from build123d import *

# Parameters (mm, degrees)
SKETCH_1_W          = 400
SKETCH_1_H          = 80
EXTRUDE_1_DEPTH     = 35
SKETCH_2_W          = 400
SKETCH_2_H          = 61
CUT_EXTRUDE_1_DEPTH = 10
CHAMFER_1_SIZE      = 5
CHAMFER_2_SIZE      = 10
CHAMFER_2_SIZE2     = 7.002075382
CHAMFER_3_SIZE      = 10
CHAMFER_3_SIZE2     = 7.002075382
CHAMFER_4_SIZE      = 10
CHAMFER_4_SIZE2     = 7.002075382
CHAMFER_5_SIZE      = 10
CHAMFER_5_SIZE2     = 7.002075382
CUT_EXTRUDE_2_REACH = 207.487
SKETCH_3_R          = 9
SKETCH_3_R_2        = 10


with BuildPart() as part:
    # 草图1 → 凸台-拉伸1 (new body)
    with BuildSketch(Plane.XY):
        Rectangle(SKETCH_1_W, SKETCH_1_H)
    extrude(amount=EXTRUDE_1_DEPTH)

    # 草图2 → 切除-拉伸1 (cut)
    with BuildSketch(Plane.XY.offset(35)):
        with Locations((0, 9.5)):
            Rectangle(SKETCH_2_W, SKETCH_2_H)
    extrude(amount=-CUT_EXTRUDE_1_DEPTH, mode=Mode.SUBTRACT)

    # 倒角1
    chamfer_1_edges = [part.edges().sort_by_distance(p)[0] for p in [
        (0, 40, 25),
        (0, 40, 0),
    ]]
    chamfer(chamfer_1_edges, length=CHAMFER_1_SIZE)

    # 倒角2
    chamfer_2_edges = [part.edges().sort_by_distance(p)[0] for p in [
        (0, -40, 35),
    ]]
    chamfer_2_side = [part.faces().sort_by_distance(p)[0] for p in [
        (0, -40, 17.5),
    ]]
    chamfer(chamfer_2_edges, length=CHAMFER_2_SIZE, length2=CHAMFER_2_SIZE2, reference=chamfer_2_side[0])

    # 倒角3
    chamfer_3_edges = [part.edges().sort_by_distance(p)[0] for p in [
        (0, -40, 0),
    ]]
    chamfer_3_side = [part.faces().sort_by_distance(p)[0] for p in [
        (0, -40, 12.5),
    ]]
    chamfer(chamfer_3_edges, length=CHAMFER_3_SIZE, length2=CHAMFER_3_SIZE2, reference=chamfer_3_side[0])

    # 倒角4
    chamfer_4_edges = [part.edges().sort_by_distance(p)[0] for p in [
        (-200, -40, 17.5),
    ]]
    chamfer_4_side = [part.faces().sort_by_distance(p)[0] for p in [
        (0, -40, 17.5),
    ]]
    chamfer(chamfer_4_edges, length=CHAMFER_4_SIZE, length2=CHAMFER_4_SIZE2, reference=chamfer_4_side[0])

    # 倒角5
    chamfer_5_edges = [part.edges().sort_by_distance(p)[0] for p in [
        (200, -40, 17.5),
    ]]
    chamfer_5_side = [part.faces().sort_by_distance(p)[0] for p in [
        (5, -40, 17.5),
    ]]
    chamfer(chamfer_5_edges, length=CHAMFER_5_SIZE, length2=CHAMFER_5_SIZE2, reference=chamfer_5_side[0])

    # 草图3 → 切除-拉伸2 (cut, up to next)
    with BuildSketch(Plane.XY.offset(25), mode=Mode.PRIVATE) as cut_extrude_2_sk1:
        with Locations((-150, 9.5)):
            Circle(SKETCH_3_R)
    cut_extrude_2_tool1 = extrude(cut_extrude_2_sk1.sketch, amount=-CUT_EXTRUDE_2_REACH, mode=Mode.PRIVATE) & part.part
    # 草图3 → 切除-拉伸2 (cut, up to next)
    with BuildSketch(Plane.XY.offset(25), mode=Mode.PRIVATE) as cut_extrude_2_sk2:
        with Locations((-100, 9.5)):
            Circle(SKETCH_3_R_2)
    cut_extrude_2_tool2 = extrude(cut_extrude_2_sk2.sketch, amount=-CUT_EXTRUDE_2_REACH, mode=Mode.PRIVATE) & part.part
    # 草图3 → 切除-拉伸2 (cut, up to next)
    with BuildSketch(Plane.XY.offset(25), mode=Mode.PRIVATE) as cut_extrude_2_sk3:
        with Locations((-50, 9.5)):
            Circle(SKETCH_3_R)
    cut_extrude_2_tool3 = extrude(cut_extrude_2_sk3.sketch, amount=-CUT_EXTRUDE_2_REACH, mode=Mode.PRIVATE) & part.part
    # 草图3 → 切除-拉伸2 (cut, up to next)
    with BuildSketch(Plane.XY.offset(25), mode=Mode.PRIVATE) as cut_extrude_2_sk4:
        with Locations((50, 9.5)):
            Circle(SKETCH_3_R)
    cut_extrude_2_tool4 = extrude(cut_extrude_2_sk4.sketch, amount=-CUT_EXTRUDE_2_REACH, mode=Mode.PRIVATE) & part.part
    # 草图3 → 切除-拉伸2 (cut, up to next)
    with BuildSketch(Plane.XY.offset(25), mode=Mode.PRIVATE) as cut_extrude_2_sk5:
        with Locations((100, 9.5)):
            Circle(SKETCH_3_R_2)
    cut_extrude_2_tool5 = extrude(cut_extrude_2_sk5.sketch, amount=-CUT_EXTRUDE_2_REACH, mode=Mode.PRIVATE) & part.part
    # 草图3 → 切除-拉伸2 (cut, up to next)
    with BuildSketch(Plane.XY.offset(25), mode=Mode.PRIVATE) as cut_extrude_2_sk6:
        with Locations((150, 9.5)):
            Circle(SKETCH_3_R)
    cut_extrude_2_tool6 = extrude(cut_extrude_2_sk6.sketch, amount=-CUT_EXTRUDE_2_REACH, mode=Mode.PRIVATE) & part.part
    add(cut_extrude_2_tool1.solids().sort_by_distance((-150, 9.5, 25))[0], mode=Mode.SUBTRACT)
    add(cut_extrude_2_tool2.solids().sort_by_distance((-100, 9.5, 25))[0], mode=Mode.SUBTRACT)
    add(cut_extrude_2_tool3.solids().sort_by_distance((-50, 9.5, 25))[0], mode=Mode.SUBTRACT)
    add(cut_extrude_2_tool4.solids().sort_by_distance((50, 9.5, 25))[0], mode=Mode.SUBTRACT)
    add(cut_extrude_2_tool5.solids().sort_by_distance((100, 9.5, 25))[0], mode=Mode.SUBTRACT)
    add(cut_extrude_2_tool6.solids().sort_by_distance((150, 9.5, 25))[0], mode=Mode.SUBTRACT)


solid = part.part
Can you work these out from the model? Positions are in its coordinate system, mm. A direction names the side the tool comes from. Round coordinates to 2 decimals unless told otherwise and drop trailing zeros. Order: outer loops, then holes, each group sorted by start corner. A loop starts at its lowest first (then second) coordinate and runs counter-clockwise, first axis right, second up. Notation, with made-up numbers: (-4.5, 40.25) - (4.5, 40.25) arc R22 cw to (4.5, 56.25) - close; hole circle Ø9 at (86, 41). An arc over 180 degrees is marked (long way). Answer in a Markdown table with one row per item.
(1) Which directions (+Z, -Z, +X, -X, +Y, -Y) give clear straight access to the entire face, cutting with the end or side of a thin tool? Please do faces 1 (the face through (196.181, -35.672, 17.255)), 2 (the face through (-3, -21, 30)).
From the geometry:
| item | result |
|---|---|
| face 1 | +Z, -Z, +X, -Y |
| face 2 | +Z, +X, -X, +Y |
(2) Suppose I cut it at D-D, the plane y = -17.5. Please give me the cut outline in (x, z), plus the area to 3 significant figures.
From the geometry:
| item | result |
|---|---|
| outline | (-200, 0) - (200, 0) - (200, 25) - (-200, 25) - close |
| area | 10,000 mm2 |
(3) If we mould it in two halves opening along X, with no side actions, what happens to faces 3 (the face through (-200, 3, 13)), 4 (the face through (-157.14, 4.02, 12.68)), 5 (the face through (92.06, 3.42, 12.68)), 6 (the face through (-2.8, -36.45, 4.93))? For each: released by +X, released by -X, zero draft, split by the parting line, or undercut.
From the geometry:
| item | result |
|---|---|
| face 3 | released by -X |
| face 4 | undercut |
| face 5 | undercut |
| face 6 | zero draft |
(4) For P1, Ø18, axis at x = -100, y = 9.5, coming from the +Z side; P2, Ø1.5, axis at x = 88, y = -13.5, coming from the +Z side; P3, Ø5, axis at x = -54.5, z = 30, coming from the +Y side; P4, Ø10, axis at x = -34, z = 29.5, coming from the +Y side, each with a flat end and sliding along its axis, tell me the tip position at first contact or that it passes through.
From the geometry:
| item | result |
|---|---|
| P1 | passes through |
| P2 | stops at z = 25 |
| P3 | stops at y = -21 |
| P4 | stops at y = 35.5 |
(5) Suppose I cut it at B-B, the plane x = -50. Please give me the cut outline in (y, z), plus the area to 3 significant figures.
From the geometry:
| item | result |
|---|---|
| outline | (-40, 10) - (-33, 0) - (0.5, 0) - (0.5, 25) - (-21, 25) - (-21, 35) - (-33, 35) - (-40, 25) - close; (18.5, 0) - (35, 0) - (40, 5) - (40, 20) - (35, 25) - (18.5, 25) - close |
| area | 1,640 mm2 |
(6) Suppose I cut it at A-A, the plane y = 9.5. Please give me the cut outline in (x, z).
From the geometry:
| item | result |
|---|---|
| outline | (-200, 0) - (-159, 0) - (-159, 25) - (-200, 25) - close; (-141, 0) - (-110, 0) - (-110, 25) - (-141, 25) - close; (-90, 0) - (-59, 0) - (-59, 25) - (-90, 25) - close; (-41, 0) - (41, 0) - (41, 25) - (-41, 25) - close; (59, 0) - (90, 0) - (90, 25) - (59, 25) - close; (110, 0) - (141, 0) - (141, 25) - (110, 25) - close; (159, 0) - (200, 0) - (200, 25) - (159, 25) - close |
(7) Please list where these lines run through material, in increasing order: L1, parallel to Y at x = -150, z = 12.5; L2, parallel to Z at x = -179, y = -9.5; L3, parallel to Y at x = -50, z = 9. Write a range as from..to.
From the geometry:
| item | result |
|---|---|
| L1 | y = -40..0.5, 18.5..40 |
| L2 | z = 0..25 |
| L3 | y = -39.3..0.5, 18.5..40 |
(8) Suppose I cut it at C-C, the plane x = 100. Please give me the cut outline in (y, z).
From the geometry:
| item | result |
|---|---|
| outline | (-40, 10) - (-33, 0) - (-0.5, 0) - (-0.5, 25) - (-21, 25) - (-21, 35) - (-33, 35) - (-40, 25) - close; (19.5, 0) - (35, 0) - (40, 5) - (40, 20) - (35, 25) - (19.5, 25) - close |
